Geometry: final body of the model. Coordinates: model frame, mm. Face numbers are marked on the shaded views. Coordinates: 2 decimals unless noted, no trailing zeros. Write each loop counter-clockwise with the first axis right and the second up, starting at its lowest first coordinate (ties: lowest second). Pieces come first, ordered by that corner, then holes. Notation, with made-up numbers: M -4.75,5.25 L 31.25,5.25 A24 ccw 31.25,25.25 Z; hole C -40,-20.5 d6. An arc over 180 degrees is marked long. Write item = value, one per line. Start each with the question number.
Item 1: Section D-D on y = -14. Output: boundary loops of the cut face in (x, z), plus the area to 3 significant figures.
Item 2: Section C-C on x = -57. Output: boundary loops of the cut face in (y, z), plus the area to 3 significant figures.
Item 3: Section A-A on y = -20.5. Output: boundary loops of the cut face in (x, z), plus the area to 3 significant figures.
Item 4: Ray query, L1, parallel to Y at x = -60, z = 14; L2, parallel to X at y = -4, z = 11; L3, parallel to Y at x = -99.5, z = 4.5. Return the intervals inside material, ascending. Write a range as [from, to].
Item 5: Section B-B on z = 19.5. Output: boundary loops of the cut face in (x, y).
Item 6: First-contact query: pin 1 Ø6 at (x, z) = (-82, 21) entering from +Y; pin 2 Ø2 at (y, z) = (-7.5, 18.5) entering from -X; pin 3 Ø1 at (x, z) = (-43, 6) entering from +Y. Flat tips, straight axial feed; report the tip coordinate or a pass-through.
Item 7: Pull-direction query (X, two-part tool) for the marked faces 1, 2 and 3; classes: +X half, -X half, draft (parallel to the pull), parting line (faces both ways), or undercut.
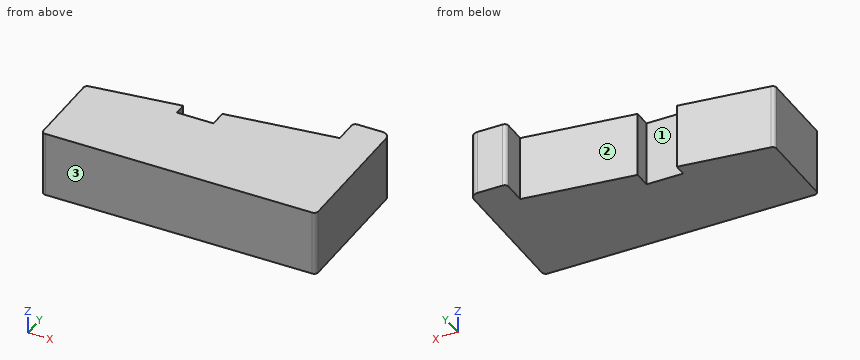
from build123d import *

# Parameters (mm, degrees)
F1_DEPTH = 25


with BuildPart() as f1:
    # F0 (on Top) → F1 (new body)
    with BuildSketch(Plane.XY):
        with BuildLine():
            ThreePointArc((-105, -53.457447), (-104.56066, -54.518107), (-103.5, -54.957447))
            Line((-103.5, -54.957447), (-56, -54.957447))
            Line((-56, -54.957447), (-1.5, -54.957447))
            ThreePointArc((-1.5, -54.957447), (-0.43934, -54.518107), (0, -53.457447))
            Line((0, -53.457447), (0, -3.957447))
            ThreePointArc((0, -3.957447), (-0.87868, -1.836126), (-3, -0.957447))
            Line((-3, -0.957447), (-12.5, -0.957447))
            ThreePointArc((-12.5, -0.957447), (-13.56066, -1.396786), (-14, -2.457447))
            Line((-14, -2.457447), (-14, -10.957447))
            Line((-14, -10.957447), (-56, -16.495908))
            Line((-56, -16.495908), (-56, -22.957447))
            Line((-56, -22.957447), (-70, -22.957447))
            Line((-70, -22.957447), (-70, -18.342062))
            Line((-70, -18.342062), (-103.696104, -22.785504))
            ThreePointArc((-103.696104, -22.785504), (-104.627865, -23.283731), (-105, -24.27263))
            Line((-105, -24.27263), (-105, -53.457447))
        make_face()
    extrude(amount=F1_DEPTH)


solid = f1.part
Responses:
q1.outline = M -37.07,0 L 0,0 L 0,25 L -37.07,25 Z
q1.area = 927 mm²
q2.outline = M -54.96,0 L -22.96,0 L -22.96,25 L -54.96,25 Z
q2.area = 800 mm²
q3.outline = M -86.36,0 L -70,0 L -70,25 L -86.36,25 Z; M -56,0 L 0,0 L 0,25 L -56,25 Z
q3.area = 1,810 mm²
q4.L1 = [-54.96, -22.96]
q4.L2 = [-14, 0]
q4.L3 = [-54.96, -22.23]
q5.outline = M -105,-53.46 A1.5 ccw -103.5,-54.96 L -1.5,-54.96 A1.5 ccw 0,-53.46 L 0,-3.96 A3 ccw -3,-0.96 L -12.5,-0.96 A1.5 ccw -14,-2.46 L -14,-10.96 L -56,-16.5 L -56,-22.96 L -70,-22.96 L -70,-18.34 L -103.7,-22.79 A1.5 ccw -105,-24.27 Z
q6.pin_1 = -19.53
q6.pin_2 = -14
q6.pin_3 = -14.72
q7.face_1 = undercut
q7.face_2 = -X half
q7.face_3 = draft
